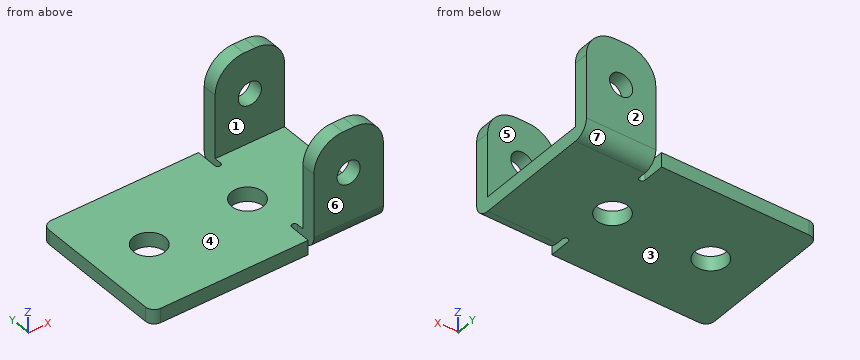
from build123d import *

# Parameters (mm, degrees)
SCHIZZO1_R                 = 2.75
BASE_FLANGIA1_DEPTH        = 2.5
BORDO_FLANGIA1_START       = -2.5
BORDO_FLANGIA1_DEPTH       = 2.5
BORDO_FLANGIA1_2_OUTLINE_W = 12
BORDO_FLANGIA1_2_OUTLINE_H = 2.5
BORDO_FLANGIA1_2_DEPTH     = 16
BORDO_FLANGIA1_START_2     = 8
BORDO_FLANGIA1_3_DEPTH     = 13
SCHIZZO12_R                = 2
TAGLIO_ESTRUSIONE1_DEPTH   = 25
TAGLIO_ESTRUSIONE2_DEPTH   = 25


with BuildPart() as part:
    # Base-Flangia1: sheet metal written as solids
    # Schizzo1 → Base-Flangia1 (new body)
    with BuildSketch(Plane.XY):
        with BuildLine():
            Line((20, -12.5), (-18.5, -12.5))
            ThreePointArc((-18.5, -12.5), (-19.560660172, -12.060660172), (-20, -11))
            Line((-20, -11), (-20, 11))
            ThreePointArc((-20, 11), (-19.560660172, 12.060660172), (-18.5, 12.5))
            Line((-18.5, 12.5), (20, 12.5))
            Line((20, 12.5), (20, -12.5))
        make_face()
        with Locations((-11, 0)):
            Circle(SCHIZZO1_R, mode=Mode.SUBTRACT)
        with Locations((6, 0)):
            Circle(SCHIZZO1_R, mode=Mode.SUBTRACT)
    extrude(amount=-BASE_FLANGIA1_DEPTH)

    # Bordo-Flangia1: read off the stored shape, not the designer's step
    # Bordo-Flangia1 outline → Bordo-Flangia1 (cut)
    with BuildSketch(Plane.XY.offset(BORDO_FLANGIA1_START)):
        with BuildLine():
            Line((8, 8.75), (8, 12.5))
            Line((8, 12.5), (7, 12.5))
            Line((7, 12.5), (7, 8.75))
            ThreePointArc((7, 8.75), (7.5, 8.25), (8, 8.75))
        make_face()
        with BuildLine():
            Line((8, -12.5), (8, -8.75))
            ThreePointArc((8, -8.75), (7.5, -8.25), (7, -8.75))
            Line((7, -8.75), (7, -12.5))
            Line((7, -12.5), (8, -12.5))
        make_face()
    extrude(amount=BORDO_FLANGIA1_DEPTH, mode=Mode.SUBTRACT)

    # Bordo-Flangia1 2 outline → Bordo-Flangia1 2 (add)
    with BuildSketch(Plane.XY):
        with Locations((14, 11.25)):
            Rectangle(BORDO_FLANGIA1_2_OUTLINE_W, BORDO_FLANGIA1_2_OUTLINE_H)
        with Locations((14, -11.25)):
            Rectangle(BORDO_FLANGIA1_2_OUTLINE_W, BORDO_FLANGIA1_2_OUTLINE_H)
    extrude(amount=BORDO_FLANGIA1_2_DEPTH)

    # Bordo-Flangia1 3 outline → Bordo-Flangia1 3 (cut)
    with BuildSketch(Plane.YZ.offset(BORDO_FLANGIA1_START_2)):
        with BuildLine():
            Line((-12.5, -2.5), (-10, -2.5))
            ThreePointArc((-10, -2.5), (-11.767766953, -1.767766953), (-12.5, 0))
            Line((-12.5, 0), (-12.5, -2.5))
        make_face()
        with BuildLine():
            ThreePointArc((12.5, 0), (11.767766953, -1.767766953), (10, -2.5))
            Line((10, -2.5), (12.5, -2.5))
            Line((12.5, -2.5), (12.5, 0))
        make_face()
    extrude(amount=BORDO_FLANGIA1_3_DEPTH, mode=Mode.SUBTRACT)

    # Schizzo12 → Taglio-Estrusione1 (cut)
    with BuildSketch(Plane.XZ.offset(12.5)):
        with Locations(Location((14, 8.5, 0), (0, 0, 270))):
            Circle(SCHIZZO12_R)
    extrude(amount=-TAGLIO_ESTRUSIONE1_DEPTH, mode=Mode.SUBTRACT)

    # Schizzo13 → Taglio-Estrusione2 (cut)
    with BuildSketch(Plane.XZ.offset(12.5)):
        with BuildLine():
            Line((8, 11), (8, 16))
            Line((8, 16), (13, 16))
            ThreePointArc((13, 16), (9.464466094, 14.535533906), (8, 11))
        make_face()
        with BuildLine():
            Line((20, 16), (20, 11))
            ThreePointArc((20, 11), (18.535533906, 14.535533906), (15, 16))
            Line((15, 16), (20, 16))
        make_face()
    extrude(amount=-TAGLIO_ESTRUSIONE2_DEPTH, mode=Mode.SUBTRACT)


solid = part.part
Source: CAD feature listing. Evaluate the final solid. Frame: model axes, mm. Face numbers are marked on the shaded views. A direction names the side the tool comes from. Give positions to 0.01 mm unless a question says otherwise; leave off trailing zeros. Write each loop counter-clockwise with the first axis right and the second up, starting at its lowest first coordinate (ties: lowest second). Pieces come first, ordered by that corner, then holes. Notation, with made-up numbers: (-39.5, 17) - (19.5, 17) arc R11 cw to (19.5, 30) - close; hole circle Ø1 at (-5.75, -11.75). An arc over 180 degrees is marked (long way). Write item = value, one per line. Start each with the question number.
Q1. Reachability of the marked faces 4, 5, 6 and 7 from +Z, -Z, +X, -X, +Y, -Y: full face, straight path, thin tool, end or side. Return the list, or none.
Q2. Cut plane D-D, the plane y = 0. Return loops of the section in (x, z).
Q3. Cut plane C-C, the plane x = 14. Return loops of the section in (y, z).
Q4. Draft query along Y for the marked faces 1, 2 and 3. Return one class per face: +Y half, -Y half, draft (parallel to the pull), parting line (faces both ways), or undercut.
Q5. Cut plane A-A, the plane x = -11. Return loops of the section in (y, z), then the cut area to 4 significant figures.
Q6. Cut plane B-B, the plane z = 8.5. Return loops of the section in (x, y), then the cut area to 3 significant figures.
Q7. Material intervals for probe 1 along X at (y, z) = (-11.5, 8.5); probe 2 along Y at (x, z) = (6, -0.6); probe 3 along Y at (x, z) = (11.5, 8.75), sorted ascending.
Q8. Pin query (flat end, axial travel): pin 1 Ø12.5 at (x, y) = (8, -0.5) entering from +Z; pin 2 Ø4.5 at (x, z) = (14, 8.5) entering from -Y; pin 3 Ø1.9 at (y, z) = (10, 4.5) entering from -X. Return the tip coordinate at first contact, or that it passes through.
Computed values:
q1.face_4 = +Z, -X
q1.face_5 = +Z, +X, -X
q1.face_6 = +Z, -Z, +X, -X, -Y
q1.face_7 = -Z, +X, +Y
q2.outline = (-20, -2.5) - (-13.75, -2.5) - (-13.75, 0) - (-20, 0) - close; (-8.25, -2.5) - (3.25, -2.5) - (3.25, 0) - (-8.25, 0) - close; (8.75, -2.5) - (20, -2.5) - (20, 0) - (8.75, 0) - close
q3.outline = (-12.5, 0) arc R2.5 ccw to (-10, -2.5) - (10, -2.5) arc R2.5 ccw to (12.5, 0) - (12.5, 6.5) - (10, 6.5) - (10, 0) - (-10, 0) - (-10, 6.5) - (-12.5, 6.5) - close; (-12.5, 10.5) - (-10, 10.5) - (-10, 16) - (-12.5, 16) - close; (10, 10.5) - (12.5, 10.5) - (12.5, 16) - (10, 16) - close
q4.face_1 = undercut
q4.face_2 = +Y half
q4.face_3 = draft
q5.outline = (-12.5, -2.5) - (-2.75, -2.5) - (-2.75, 0) - (-12.5, 0) - close; (2.75, -2.5) - (12.5, -2.5) - (12.5, 0) - (2.75, 0) - close
q5.area = 48.75 mm²
q6.outline = (8, -12.5) - (12, -12.5) - (12, -10) - (8, -10) - close; (8, 10) - (12, 10) - (12, 12.5) - (8, 12.5) - close; (16, -12.5) - (20, -12.5) - (20, -10) - (16, -10) - close; (16, 10) - (20, 10) - (20, 12.5) - (16, 12.5) - close
q6.area = 40.0 mm²
q7.probe_1 = 8 to 12, 16 to 20
q7.probe_2 = -12.5 to -2.75, 2.75 to 12.5
q7.probe_3 = -12.5 to -10, 10 to 12.5
q8.pin_1 = 0
q8.pin_2 = -12.5
q8.pin_3 = 8
